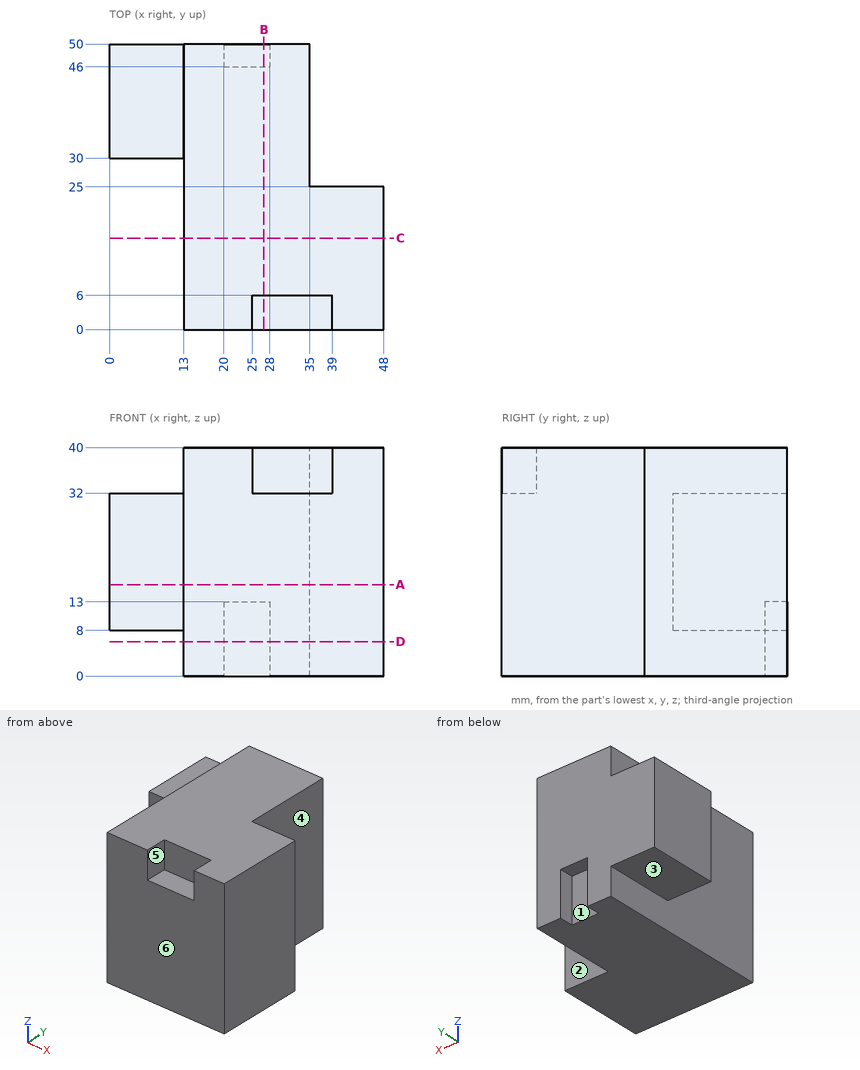
Print and shaded views of the part. All mm, measured from the part's lowest x, y and z. A direction names the side the tool comes from. Round coordinates to 2 decimals unless told otherwise and drop trailing zeros. Write each loop counter-clockwise with the first axis right and the second up, starting at its lowest first coordinate (ties: lowest second). Pieces come first, ordered by that corner, then holes. Notation, with made-up numbers: M 75.5,64 L 127.5,64 A11 cw 127.5,75 Z; hole C -16.75,33 d11. An arc over 180 degrees is marked long. Use a Markdown table: item, result. Add a question column.
1. Slice it at C-C on y = 16. Give the cut face in (x, z), then the cut area to 3 significant figures.
2. Pull direction X, two halves, no side cores. Call the marked faces 4, 5 and 6: released by +X, released by -X, zero draft, split by the parting line, or undercut.
3. Flat gauge pins, fed straight in: P1, Ø12.5, axis at y = 31.5, z = 16.5, coming from the +X side; P2, Ø4, axis at x = 32, z = 36.5, coming from the -Y side; P3, Ø8, axis at y = 14, z = 20, coming from the -X side. Where does each tip first touch, or does it go through?
4. Slice it at A-A on z = 16. Give the cut face in (x, y).
5. Slice it at D-D on z = 6. Give the cut face in (x, y), then the cut area to 3 significant figures.
6. Drill centre lines: probe 1 along X at (y, z) = (47.5, 17); probe 2 along X at (y, z) = (23.5, 20); probe 3 along Y at (x, z) = (4, 26). Where is each one in solid material? Low to high.
7. 3-axis set-ups, long thin cutter, end or side, ignore diameter. For the marked faces 1, 2 and 3: which of +Z, -Z, +X, -X, +Y, -Y reach the whole face in a straight line?
8. Slice it at B-B on x = 27. Give the cut face in (y, z), then the cut area to 3 significant figures.
Reply:
| question | item | result |
|---|---|---|
| 1 | outline | M 13,0 L 48,0 L 48,40 L 13,40 Z |
| 1 | area | 1,400 mm^2 |
| 2 | face 4 | released by +X |
| 2 | face 5 | undercut |
| 2 | face 6 | zero draft |
| 3 | P1 | stops at x = 35 |
| 3 | P2 | stops at y = 6 |
| 3 | P3 | stops at x = 13 |
| 4 | outline | M 0,30 L 13,30 L 13,0 L 48,0 L 48,25 L 35,25 L 35,50 L 0,50 Z |
| 5 | outline | M 13,0 L 48,0 L 48,25 L 35,25 L 35,50 L 28,50 L 28,46 L 20,46 L 20,50 L 13,50 Z |
| 5 | area | 1,390 mm^2 |
| 6 | probe 1 | x = 0 to 35 |
| 6 | probe 2 | x = 13 to 48 |
| 6 | probe 3 | y = 30 to 50 |
| 7 | face 1 | -Z, +Y |
| 7 | face 2 | +Z, -Z, +X, +Y |
| 7 | face 3 | -Z, -X, +Y, -Y |
| 8 | outline | M 0,0 L 46,0 L 46,13 L 50,13 L 50,40 L 6,40 L 6,32 L 0,32 Z |
| 8 | area | 1,900 mm^2 |
